Here's how the part is built. I have some questions about the finished solid (model axes, mm). A direction names the side the tool comes from. Round coordinates to 2 decimals unless told otherwise and drop trailing zeros. Loops run counter-clockwise (first coordinate to the right, second up) from the corner with the lowest first, then second, coordinate; pieces in that order, holes last. Notation, with made-up numbers: M -35,-11 L 10,-11 A22 cw 10,25 Z; hole C -12,41.5 d11. An arc over 180 degrees is marked long. Write each question's results on one line, items separated by ' | '. Start each with the question number.
```python
from build123d import *

# Parameters (mm, degrees)
SKETCH1_R                = 16
SKETCH1_R_2              = 11
BOSS_EXTRUDE1_DEPTH      = 7
BOSS_EXTRUDE2_DEPTH      = 10
BOSS_EXTRUDE2_DEPTH_BACK = 10
SKETCH3_W                = 13
SKETCH3_H                = 13
CUT_EXTRUDE1_DEPTH       = 26
BOSS_EXTRUDE5_START      = 6.5
SKETCH8_R                = 16
SKETCH8_R_2              = 8
BOSS_EXTRUDE5_DEPTH      = 6.5
SKETCH9_R                = 1
BOSS_EXTRUDE6_DEPTH      = 20
CUT_EXTRUDE3_DEPTH       = 5
CUT_EXTRUDE3_DEPTH_BACK  = 5
BOSS_EXTRUDE7_START      = -8.5
BOSS_EXTRUDE7_DEPTH      = 8.5
CUT_EXTRUDE4_START       = -13.5
SKETCH12_R               = 1.75
CUT_EXTRUDE4_DEPTH       = 13.5
SKETCH13_R               = 4.75
CUT_EXTRUDE5_DEPTH       = 5
CUT_EXTRUDE6_REACH       = 59.783
SKETCH14_R               = 2.5


with BuildPart() as part:
    # Sketch1 → Boss-Extrude1 (new body)
    with BuildSketch(Plane.XY):
        Circle(SKETCH1_R)
        Circle(SKETCH1_R_2, mode=Mode.SUBTRACT)
    extrude(amount=BOSS_EXTRUDE1_DEPTH)

    # Sketch2 → Boss-Extrude2 (add, two sides: drawn at the far end of the back side and taken through both)
    with BuildSketch(Plane.XY.offset(3.5).offset(-BOSS_EXTRUDE2_DEPTH_BACK)):
        with BuildLine():
            Line((-12.233132214, 10.312636725), (-44.939361172, 6.978812037))
            Line((-44.939361172, 6.978812037), (-42.607001327, -15.902623617))
            Line((-42.607001327, -15.902623617), (-9.900772369, -12.568798928))
            ThreePointArc((-9.900772369, -12.568798928), (-15.917520454, -1.622511196), (-12.233132214, 10.312636725))
        make_face()
    extrude(amount=BOSS_EXTRUDE2_DEPTH + BOSS_EXTRUDE2_DEPTH_BACK)

    # Sketch3 → Cut-Extrude1 (cut)
    with BuildSketch(Plane(origin=(-43.77318125, -4.46190579, 0), x_dir=(0, 0, 1), z_dir=(-0.9948450284027645, -0.10140694977319323, 0))):
        with Locations((3.5, 0)):
            Rectangle(SKETCH3_W, SKETCH3_H)
    extrude(amount=-CUT_EXTRUDE1_DEPTH, mode=Mode.SUBTRACT)

    # Sketch8 → Boss-Extrude5 (add)
    with BuildSketch(Plane(origin=(0, 0, 0), x_dir=(-1, 0, 0), z_dir=(0, 0, -1)).offset(BOSS_EXTRUDE5_START)):
        Circle(SKETCH8_R)
        with Locations(Location((0, 0, 0), (0, 0, 180))):
            Circle(SKETCH8_R_2, mode=Mode.SUBTRACT)
    extrude(amount=-BOSS_EXTRUDE5_DEPTH)

    # Sketch9 → Boss-Extrude6 (add)
    with BuildSketch(Plane(origin=(0, 0, -6.5), x_dir=(-1, 0, 0), z_dir=(0, 0, -1))):
        with BuildLine():
            Line((42.607001327, -15.902623617), (32.658551043, -14.888554119))
            Line((32.658551043, -14.888554119), (31.973720208, -21.607033999))
            ThreePointArc((31.973720208, -21.607033999), (36.440910601, -27.08829389), (41.922170492, -22.621103497))
            Line((41.922170492, -22.621103497), (42.607001327, -15.902623617))
        make_face()
        with Locations((36.94794535, -22.114068748)):
            Circle(SKETCH9_R, mode=Mode.SUBTRACT)
    extrude(amount=-BOSS_EXTRUDE6_DEPTH)

    # Sketch10 → Cut-Extrude3 (cut, two sides: drawn at the far end of the back side and taken through both)
    with BuildSketch(Plane.XY.offset(3.5).offset(-CUT_EXTRUDE3_DEPTH_BACK)):
        with BuildLine():
            Line((-32.658551043, -14.888554119), (-42.607001327, -15.902623617))
            Line((-42.607001327, -15.902623617), (-41.922170492, -22.621103497))
            ThreePointArc((-41.922170492, -22.621103497), (-36.440910601, -27.08829389), (-31.973720208, -21.607033999))
            Line((-31.973720208, -21.607033999), (-32.658551043, -14.888554119))
        make_face()
    extrude(amount=CUT_EXTRUDE3_DEPTH + CUT_EXTRUDE3_DEPTH_BACK, mode=Mode.SUBTRACT)

    # Sketch11 → Boss-Extrude7 (add)
    with BuildSketch(Plane.XY.offset(7).offset(BOSS_EXTRUDE7_START)):
        with BuildLine():
            ThreePointArc((6.224175029, -14.739730161), (2.104194208, -20.643034339), (-3.12215228, -15.692423813))
            ThreePointArc((-3.12215228, -15.692423813), (1.622511196, -15.917520454), (6.224175029, -14.739730161))
        make_face()
    boss_extrude7 = extrude(amount=BOSS_EXTRUDE7_DEPTH)

    # Sketch12 → Cut-Extrude4 (cut)
    with BuildSketch(Plane.XY.offset(7).offset(CUT_EXTRUDE4_START)):
        with Locations((1.622511196, -15.917520454)):
            Circle(SKETCH12_R)
    cut_extrude4 = extrude(amount=CUT_EXTRUDE4_DEPTH, mode=Mode.SUBTRACT)

    # Mirror1: Boss-Extrude7, Cut-Extrude4 across plane
    add(boss_extrude7.mirror(Plane(origin=(0, 0, 0), x_dir=(0, 0, 1), z_dir=(0.10140694977319331, -0.9948450284027645, 0))))
    add(cut_extrude4.mirror(Plane(origin=(0, 0, 0), x_dir=(0, 0, 1), z_dir=(0.10140694977319331, -0.9948450284027645, 0))), mode=Mode.SUBTRACT)

    # Sketch13 → Cut-Extrude5 (cut)
    with BuildSketch(Plane(origin=(0, 0, -6.5), x_dir=(-1, 0, 0), z_dir=(0, 0, -1))):
        with Locations((-1.622511196, -15.917520454)):
            Circle(SKETCH13_R)
        with Locations((1.622511196, 15.917520454)):
            Circle(SKETCH13_R)
    extrude(amount=-CUT_EXTRUDE5_DEPTH, mode=Mode.SUBTRACT)

    # Cut-Extrude6: up to this face of the body (flat: up to its plane)
    cut_extrude6_end = Plane(part.part.faces().sort_by_distance((-28.586246693, 8.645724381, 3.5))[0])
    # Sketch14 → Cut-Extrude6 (cut, up to the picked face)
    with BuildSketch(Plane(origin=(1.166179922, -11.440717827, 0), x_dir=(0.9948450284027645, 0.1014069497731933, 0), z_dir=(0.1014069497731933, -0.9948450284027645, 0)), mode=Mode.PRIVATE) as cut_extrude6_sk1:
        with Locations((-39, 3.5)):
            Circle(SKETCH14_R)
    cut_extrude6_tool1 = split(extrude(cut_extrude6_sk1.sketch, amount=-CUT_EXTRUDE6_REACH, mode=Mode.PRIVATE), bisect_by=cut_extrude6_end, keep=Keep.BOTH, mode=Mode.PRIVATE)
    # Sketch14 → Cut-Extrude6 (cut, up to the picked face)
    with BuildSketch(Plane(origin=(1.166179922, -11.440717827, 0), x_dir=(0.9948450284027645, 0.1014069497731933, 0), z_dir=(0.1014069497731933, -0.9948450284027645, 0)), mode=Mode.PRIVATE) as cut_extrude6_sk2:
        with Locations((-23.5, 3.5)):
            Circle(SKETCH14_R)
    cut_extrude6_tool2 = split(extrude(cut_extrude6_sk2.sketch, amount=-CUT_EXTRUDE6_REACH, mode=Mode.PRIVATE), bisect_by=cut_extrude6_end, keep=Keep.BOTH, mode=Mode.PRIVATE)
    add(cut_extrude6_tool1.solids().sort_by(Axis((-37.632776, -15.395589, 3.5), (-0.1014069497731933, 0.9948450284027645, 0)))[0], mode=Mode.SUBTRACT)
    add(cut_extrude6_tool2.solids().sort_by(Axis((-22.212678, -13.823781, 3.5), (-0.1014069497731933, 0.9948450284027645, 0)))[0], mode=Mode.SUBTRACT)


solid = part.part
```
Item 1: I'm going to push flat-ended pins straight in: pin 1 (10 mm diameter, centred on y = 6.5, z = 6.5, fed in from +X); pin 2 (1.8 mm diameter, centred on x = -36.95, y = -22.11, fed in from -Z); pin 3 (4 mm diameter, centred on y = -2.5, z = 9.5, fed in from -X); pin 4 (1.5 mm diameter, centred on y = 11, z = -4.5, fed in from +X). Where does each tip first touch, or does it pass through?
Item 2: If we section it at C-C on x = 5.5: Please give me the cut outline in (y, z).
Item 3: I need wall thicknesses on L1, parallel to Y at x = -2.5, z = -1; L2, parallel to Y at x = -28, z = 9.75; L3, parallel to Y at x = -32.5, z = 6.75. Which ranges of each line are inside material? Lowest first, please.
Item 4: If we section it at D-D on y = 12: Please give me the cut outline in (x, z), and give its area (3 significant figures).
Item 5: If we mould it in two halves opening along X, with no side actions, what happens to faces 1 (the face through (-30.36, -9.63, 3.41)), 2 (the face through (-36.332, -27.076, -4.035)), 3 (the face through (-2, 14, -1.5))? For each: released by +X, released by -X, zero draft, split by the parting line, or undercut.
Item 6: If we section it at B-B on y = 0: Please give me the cut outline in (x, z), and give its area (3 significant figures).
Item 7: If we section it at A-A on z = 4.5: Count the separate pieces of the cut face and the enclosed holes in it, and give its area (3 significant figures).
Item 8: Which directions (+Z, -Z, +X, -X, +Y, -Y) give clear straight access to the entire face, cutting with the end or side of a thin tool? Please do faces 4 (the face through (-1.047, 11.203, -4.035)), 5 (the face through (1.047, -11.203, -4.035)), 6 (the face through (-17.916, -1.735, 3.409)), 7 (the face through (-2.38, -10.74, 3.45)), 8 (the face through (-21, -5, -6.5)).
Numbers:
1) pin 1: x = 15.93 | pin 2: through | pin 3: x = -44.17 | pin 4: x = 12.29
2) outline: M -18.66,-1.5 L -13.17,-1.5 L -13.17,-6.5 L -5.81,-6.5 L -5.81,0 L -9.53,0 L -9.53,7 L -18.66,7 Z; M 5.81,-6.5 L 15.02,-6.5 L 15.02,7 L 9.53,7 L 9.53,0 L 5.81,0 Z
3) L1: -18.28 to -7.6, 7.6 to 14.4, 17.43 to 20.59 | L2: -14.41 to -9.39, 3.68 to 8.71 | L3: -14.87 to -9.85, 3.22 to 8.25
4) outline: M -10.58,-6.5 L -4.31,-6.5 L -4.31,-1.5 L 1.06,-1.5 L 1.06,-6.5 L 10.58,-6.5 L 10.58,7 L -10.58,7 Z | area: 259 mm²
5) face 1: released by -X | face 2: split by the parting line | face 3: undercut
6) outline: M -44.23,-6.5 L -8,-6.5 L -8,0 L -11,0 L -11,7 L -16,7 L -16,13.5 L -44.23,13.5 L -44.23,10 L -18.09,10 L -18.09,-3 L -44.23,-3 Z; M 8,-6.5 L 16,-6.5 L 16,7 L 11,7 L 11,0 L 8,0 Z | area: 399 mm²
7) separate pieces: 5 | enclosed holes: 3 | area: 729 mm²
8) face 4: -Z, +Y | face 5: -Z, -Y | face 6: none | face 7: +Z | face 8: -Z, +X, -X, +Y, -Y
